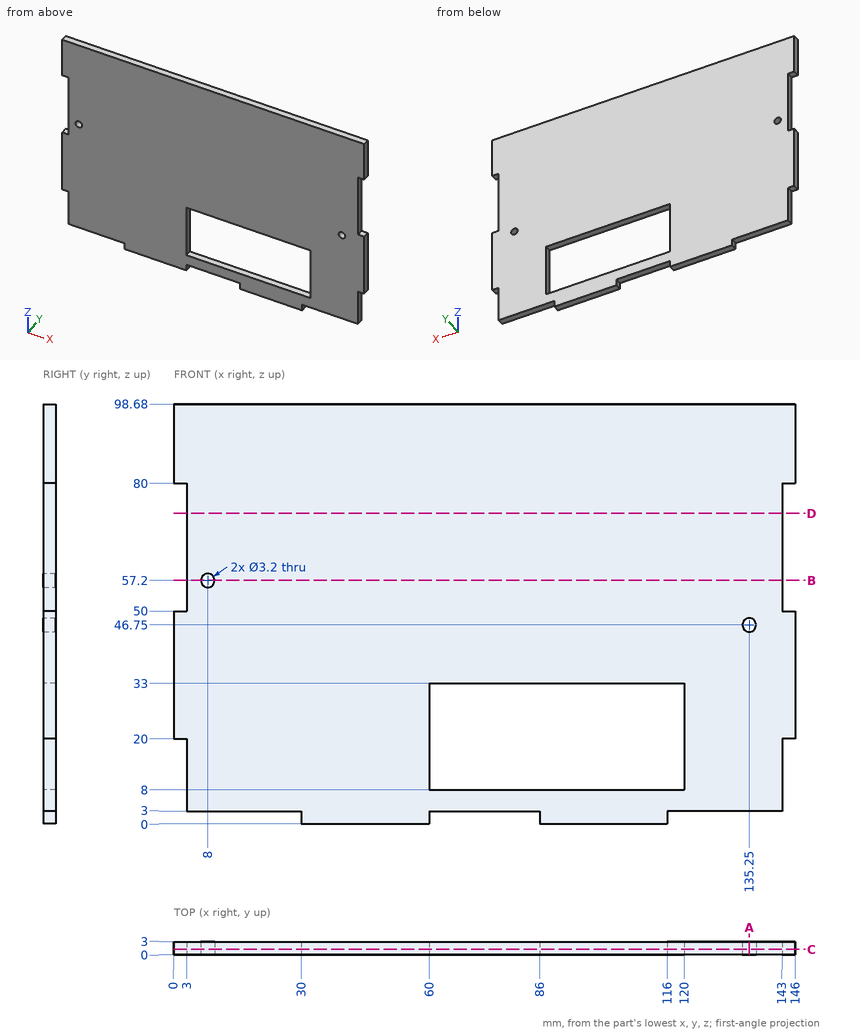
Could you check a few things on this drawing? It's one solid part, dimensions in mm from its lowest x, y, z. Give positions to 0.01 mm unless a question says otherwise; leave off trailing zeros. Order: outer loops, then holes, each group sorted by start corner. A loop starts at its lowest first (then second) coordinate and runs counter-clockwise, first axis right, second up. Notation, with made-up numbers: (45, 11) - (58, 11) arc R6 ccw to (58, 19) - close; hole circle Ø9 at (-17, -6). An arc over 180 degrees is marked (long way). One line per item, written item: value. Start each with the question number.
1. If I drill on probe 1 along X at (y, z) = (2, 57.2); probe 2 along Z at (x, y) = (111.5, 1.1); probe 3 along Z at (x, y) = (135.25, 2.3), over which ranges is the centre line in solid material (lowest first)?
2. Imagine slicing it at C-C on y = 1.25. Give the number of separate pieces and of enclosed holes in the cut face, plus the area to 3 significant figures.
3. For P1, Ø0.9, axis at y = 1.5, z = 13, coming from the +X side; P2, Ø2.5, axis at x = 135.25, z = 46.75, coming from the +Y side; P3, Ø1.5, axis at y = 1, z = 1, coming from the -X side; P4, Ø1.5, axis at x = 67.5, y = 1.5, coming from the -Z side, each with a flat end and sliding along its axis, tell me the tip position at first contact or that it passes through.
4. Imagine slicing it at B-B on z = 57.2. List the corners of the cut face in (x, y) for me.
5. Imagine slicing it at D-D on z = 73. List the corners of the cut face in (x, y) for me, plus the area to 3 significant figures.
6. Imagine slicing it at A-A on x = 135.25. List the corners of the cut face in (y, z) for me, plus the area to 3 significant figures.
Values:
1. probe 1: 3 to 6.4, 9.6 to 143
1. probe 2: 0 to 8, 33 to 98.68
1. probe 3: 3 to 45.15, 48.35 to 98.68
2. separate pieces: 1
2. enclosed holes: 3
2. area: 12,400 mm²
3. P1: x = 143
3. P2: through
3. P3: x = 30
3. P4: z = 3
4. outline: (3, 0) - (6.4, 0) - (6.4, 3) - (3, 3) - close; (9.6, 0) - (143, 0) - (143, 3) - (9.6, 3) - close
5. outline: (3, 0) - (143, 0) - (143, 3) - (3, 3) - close
5. area: 420 mm²
6. outline: (0, 3) - (3, 3) - (3, 45.15) - (0, 45.15) - close; (0, 48.35) - (3, 48.35) - (3, 98.68) - (0, 98.68) - close
6. area: 277 mm²
